from build123d import *

# Parameters (mm, degrees)
SKETCH2_W           = 41
SKETCH2_H           = 41
BOSS_EXTRUDE1_DEPTH = 2
SKETCH3_R           = 2
CUT_EXTRUDE1_DEPTH  = 30.060282173
SKETCH4_R           = 7.5
CUT_EXTRUDE2_DEPTH  = 30.060282173
SKETCH5_W           = 25
SKETCH5_H           = 25
CUT_EXTRUDE3_DEPTH  = 1
CUT_EXTRUDE4_DEPTH  = 30.060282173
SKETCH7_R           = 2
CUT_EXTRUDE5_DEPTH  = 30.060282173
SKETCH8_W           = 25
SKETCH8_H           = 8
SKETCH8_H_2         = 7.957817611
BOSS_EXTRUDE2_DEPTH = 3.5
SKETCH9_R           = 2
CUT_EXTRUDE6_DEPTH  = 30.508473359
BOSS_EXTRUDE3_START = 3.5
SKETCH10_R          = 2
BOSS_EXTRUDE3_DEPTH = 3.5
SKETCH11_R          = 3.5
CUT_EXTRUDE7_DEPTH  = 3.5
SKETCH12_W          = 8
SKETCH12_H          = 2
BOSS_EXTRUDE4_DEPTH = 3.5
SKETCH13_R          = 3.5
CUT_EXTRUDE8_DEPTH  = 3.5
SKETCH14_R          = 3.5
SKETCH14_R_2        = 2
BOSS_EXTRUDE5_DEPTH = 3
SKETCH15_W          = 16
SKETCH15_H          = 8.042182389
SKETCH15_R          = 2
SKETCH15_H_2        = 8
BOSS_EXTRUDE6_DEPTH = 4
SKETCH16_W          = 8
SKETCH16_H          = 25
CUT_EXTRUDE9_DEPTH  = 3.5
SKETCH18_W          = 32.514718626
SKETCH18_H          = 41
CUT_EXTRUDE10_DEPTH = 4
CUT_EXTRUDE12_DEPTH = 30.508473359


with BuildPart() as part:
    # Sketch2 → Boss-Extrude1 (new body)
    with BuildSketch(Plane(origin=(0, 0, 0), x_dir=(1, 0, 0), z_dir=(0, 1, 0))):
        Rectangle(SKETCH2_W, SKETCH2_H)
    extrude(amount=BOSS_EXTRUDE1_DEPTH)

    # Sketch3 → Cut-Extrude1 (cut, through all)
    with BuildSketch(Plane.XZ):
        with Locations(Location((-7.943181907, 8.037155044, 0), (0, 0, 270))):
            Circle(SKETCH3_R)
        with Locations(Location((8.037155044, 7.943181907, 0), (0, 0, 270))):
            Circle(SKETCH3_R)
        with Locations(Location((7.943181907, -8.037155044, 0), (0, 0, 270))):
            Circle(SKETCH3_R)
        with Locations(Location((-8.037155044, -7.943181907, 0), (0, 0, 270))):
            Circle(SKETCH3_R)
    extrude(amount=-CUT_EXTRUDE1_DEPTH, mode=Mode.SUBTRACT)

    # Sketch4 → Cut-Extrude2 (cut, through all)
    with BuildSketch(Plane(origin=(0, 2, 0), x_dir=(1, 0, 0), z_dir=(0, 1, 0))):
        with Locations(Location((0, 0, 0), (0, 0, 270))):
            Circle(SKETCH4_R)
    extrude(amount=-CUT_EXTRUDE2_DEPTH, mode=Mode.SUBTRACT)

    # Sketch5 → Cut-Extrude3 (cut)
    with BuildSketch(Plane.XZ):
        Rectangle(SKETCH5_W, SKETCH5_H)
    extrude(amount=-CUT_EXTRUDE3_DEPTH, mode=Mode.SUBTRACT)

    # Sketch6 → Cut-Extrude4 (cut, through all)
    with BuildSketch(Plane(origin=(0, 2, 0), x_dir=(1, 0, 0), z_dir=(0, 1, 0))):
        Polygon((-20.5, 16.257359313), (-16.257359313, 20.5), (-20.5, 20.5), align=None)
        Polygon((16.257359313, 20.5), (20.5, 16.257359313), (20.5, 20.5), align=None)
        Polygon((20.5, -16.257359313), (16.257359313, -20.5), (20.5, -20.5), align=None)
        Polygon((-16.257359313, -20.5), (-20.5, -16.257359313), (-20.5, -20.5), align=None)
    extrude(amount=-CUT_EXTRUDE4_DEPTH, mode=Mode.SUBTRACT)

    # Sketch7 → Cut-Extrude5 (cut, through all)
    with BuildSketch(Plane.XZ):
        with Locations(Location((-15.5, 15.5, 0), (0, 0, 270))):
            Circle(SKETCH7_R)
        with Locations(Location((15.5, 15.5, 0), (0, 0, 270))):
            Circle(SKETCH7_R)
        with Locations(Location((15.5, -15.5, 0), (0, 0, 270))):
            Circle(SKETCH7_R)
        with Locations(Location((-15.5, -15.5, 0), (0, 0, 270))):
            Circle(SKETCH7_R)
    extrude(amount=-CUT_EXTRUDE5_DEPTH, mode=Mode.SUBTRACT)

    # Sketch8 → Boss-Extrude2 (add)
    with BuildSketch(Plane.XZ):
        with Locations((0, 16.5)):
            Rectangle(SKETCH8_W, SKETCH8_H)
        with Locations((0, -16.478908806)):
            Rectangle(SKETCH8_W, SKETCH8_H_2)
    extrude(amount=BOSS_EXTRUDE2_DEPTH)

    # Sketch9 → Cut-Extrude6 (cut, through all)
    with BuildSketch(Plane.XZ.offset(3.5)):
        with Locations(Location((0, 16.5, 0), (0, 0, 270))):
            Circle(SKETCH9_R)
        with Locations(Location((0, -16.478908806, 0), (0, 0, 270))):
            Circle(SKETCH9_R)
    extrude(amount=-CUT_EXTRUDE6_DEPTH, mode=Mode.SUBTRACT)

    # Sketch10 → Boss-Extrude3 (add)
    # profile 1 of 3: a face of its own
    with BuildSketch(Plane.XZ.offset(BOSS_EXTRUDE3_START)):
        Polygon((-20.5, 16.257359313), (-20.5, 12.5), (-12.5, 12.5), (-12.5, 20.5), (-16.257359313, 20.5), align=None)
        with Locations(Location((-15.5, 15.5, 0), (0, 0, 270))):
            Circle(SKETCH10_R, mode=Mode.SUBTRACT)
    # profile 2 of 3: a face of its own
    with BuildSketch(Plane.XZ.offset(BOSS_EXTRUDE3_START)):
        Polygon((12.5, 12.5), (20.5, 12.5), (20.5, 16.257359313), (16.257359313, 20.5), (12.5, 20.5), align=None)
        with Locations(Location((15.5, 15.5, 0), (0, 0, 270))):
            Circle(SKETCH10_R, mode=Mode.SUBTRACT)
    # profile 3 of 3: a face of its own
    with BuildSketch(Plane.XZ.offset(BOSS_EXTRUDE3_START)):
        Polygon((-20.5, -12.5), (-20.5, -16.257359313), (-16.257359313, -20.5), (16.257359313, -20.5), (20.5, -16.257359313), (20.5, -12.5), (12.5, -12.5), (12.5, -20.457817611), (-12.5, -20.457817611), (-12.5, -12.5), align=None)
        with Locations(Location((-15.5, -15.5, 0), (0, 0, 270))):
            Circle(SKETCH10_R, mode=Mode.SUBTRACT)
        with Locations(Location((15.5, -15.5, 0), (0, 0, 270))):
            Circle(SKETCH10_R, mode=Mode.SUBTRACT)
    extrude(amount=-BOSS_EXTRUDE3_DEPTH)

    # Sketch11 → Cut-Extrude7 (cut)
    with BuildSketch(Plane(origin=(0, 2, 0), x_dir=(1, 0, 0), z_dir=(0, 1, 0))):
        with Locations(Location((-15.5, 15.5, 0), (0, 0, 270))):
            Circle(SKETCH11_R)
        with Locations(Location((15.5, 15.5, 0), (0, 0, 270))):
            Circle(SKETCH11_R)
        with Locations(Location((15.5, -15.5, 0), (0, 0, 270))):
            Circle(SKETCH11_R)
        with Locations(Location((-15.5, -15.5, 0), (0, 0, 270))):
            Circle(SKETCH11_R)
    extrude(amount=-CUT_EXTRUDE7_DEPTH, mode=Mode.SUBTRACT)

    # Sketch12 → Boss-Extrude4 (add)
    with BuildSketch(Plane.XZ):
        with Locations((-16.5, -11.5)):
            Rectangle(SKETCH12_W, SKETCH12_H)
        with Locations((-16.5, 11.5)):
            Rectangle(SKETCH12_W, SKETCH12_H)
        with Locations((16.5, -11.5)):
            Rectangle(SKETCH12_W, SKETCH12_H)
        with Locations((16.5, 11.5)):
            Rectangle(SKETCH12_W, SKETCH12_H)
    extrude(amount=BOSS_EXTRUDE4_DEPTH)

    # Sketch13 → Cut-Extrude8 (cut)
    with BuildSketch(Plane(origin=(0, 2, 0), x_dir=(1, 0, 0), z_dir=(0, 1, 0))):
        with Locations(Location((-15.5, 15.5, 0), (0, 0, 270))):
            Circle(SKETCH13_R)
        with Locations(Location((15.5, 15.5, 0), (0, 0, 270))):
            Circle(SKETCH13_R)
        with Locations(Location((15.5, -15.5, 0), (0, 0, 270))):
            Circle(SKETCH13_R)
        with Locations(Location((-15.5, -15.5, 0), (0, 0, 270))):
            Circle(SKETCH13_R)
    extrude(amount=-CUT_EXTRUDE8_DEPTH, mode=Mode.SUBTRACT)

    # Sketch14 → Boss-Extrude5 (add)
    # profile 1 of 4: a face of its own
    with BuildSketch(Plane(origin=(0, -1.5, 0), x_dir=(1, 0, 0), z_dir=(0, 1, 0))):
        with Locations(Location((-15.5, -15.5, 0), (0, 0, 270))):
            Circle(SKETCH14_R)
        with Locations(Location((-15.5, -15.5, 0), (0, 0, 90))):
            Circle(SKETCH14_R_2, mode=Mode.SUBTRACT)
    # profile 2 of 4: a face of its own
    with BuildSketch(Plane(origin=(0, -1.5, 0), x_dir=(1, 0, 0), z_dir=(0, 1, 0))):
        with Locations(Location((-15.5, 15.5, 0), (0, 0, 270))):
            Circle(SKETCH14_R)
        with Locations(Location((-15.5, 15.5, 0), (0, 0, 90))):
            Circle(SKETCH14_R_2, mode=Mode.SUBTRACT)
    # profile 3 of 4: a face of its own
    with BuildSketch(Plane(origin=(0, -1.5, 0), x_dir=(1, 0, 0), z_dir=(0, 1, 0))):
        with Locations(Location((15.5, 15.5, 0), (0, 0, 270))):
            Circle(SKETCH14_R)
        with Locations(Location((15.5, 15.5, 0), (0, 0, 90))):
            Circle(SKETCH14_R_2, mode=Mode.SUBTRACT)
    # profile 4 of 4: a face of its own
    with BuildSketch(Plane(origin=(0, -1.5, 0), x_dir=(1, 0, 0), z_dir=(0, 1, 0))):
        with Locations(Location((15.5, -15.5, 0), (0, 0, 270))):
            Circle(SKETCH14_R)
        with Locations(Location((15.5, -15.5, 0), (0, 0, 90))):
            Circle(SKETCH14_R_2, mode=Mode.SUBTRACT)
    extrude(amount=BOSS_EXTRUDE5_DEPTH)

    # Sketch15 → Boss-Extrude6 (add)
    # profile 1 of 2: a face of its own
    with BuildSketch(Plane(origin=(0, 2, 0), x_dir=(1, 0, 0), z_dir=(0, 1, 0))):
        with Locations((0, 16.478908806)):
            Rectangle(SKETCH15_W, SKETCH15_H)
        with Locations(Location((0, 16.478908806, 0), (0, 0, 90))):
            Circle(SKETCH15_R, mode=Mode.SUBTRACT)
    # profile 2 of 2: a face of its own
    with BuildSketch(Plane(origin=(0, 2, 0), x_dir=(1, 0, 0), z_dir=(0, 1, 0))):
        with Locations((0, -16.5)):
            Rectangle(SKETCH15_W, SKETCH15_H_2)
        with Locations(Location((0, -16.478908806, 0), (0, 0, 90))):
            Circle(SKETCH15_R, mode=Mode.SUBTRACT)
    extrude(amount=BOSS_EXTRUDE6_DEPTH)

    # Sketch16 → Cut-Extrude9 (cut)
    with BuildSketch(Plane.XZ.offset(3.5)):
        with Locations((-16.5, 0)):
            Rectangle(SKETCH16_W, SKETCH16_H)
        with Locations((16.5, 0)):
            Rectangle(SKETCH16_W, SKETCH16_H)
    extrude(amount=-CUT_EXTRUDE9_DEPTH, mode=Mode.SUBTRACT)

    # Sketch18 → Cut-Extrude10 (cut)
    with BuildSketch(Plane(origin=(0, 6, 0), x_dir=(1, 0, 0), z_dir=(0, 1, 0))):
        Rectangle(SKETCH18_W, SKETCH18_H)
    extrude(amount=-CUT_EXTRUDE10_DEPTH, mode=Mode.SUBTRACT)

    # Sketch19 → Cut-Extrude12 (cut, through all)
    with BuildSketch(Plane(origin=(0, 2, 0), x_dir=(1, 0, 0), z_dir=(0, 1, 0))):
        Polygon((-12, 20.5), (-12, -20.5), (-16.257359313, -20.5), (-20.5, -16.257359313), (-20.5, 16.257359313), (-16.257359313, 20.5), align=None)
    extrude(amount=-CUT_EXTRUDE12_DEPTH, mode=Mode.SUBTRACT)


solid = part.part
Input: part model. Units: mm. Frame: model coordinates. A direction names the side the tool comes from. Give positions to 0.01 mm unless a question says otherwise; leave off trailing zeros. Order: outer loops, then holes, each group sorted by start corner. A loop starts at its lowest first (then second) coordinate and runs counter-clockwise, first axis right, second up.
Q1. Ray query, probe 1 along X at (y, z) = (1.65, 8); probe 2 along Z at (x, y) = (4, 0.8); probe 3 along X at (y, z) = (-1.45, 15.5). Return the intervals inside material, ascending.
Checked values:
probe 1: x = -12 to -9.94, -5.94 to 6.04, 10.04 to 20.5
probe 2: z = -20.5 to -12.5, 12.5 to 20.5
probe 3: x = -12 to -1.73, 1.73 to 13.5, 17.5 to 20.5
Q2. Section B-B on y = -0.6. Output: boundary loops of the cut face in (x, z).
Checked values:
outline: (-12, -20.5) - (16.26, -20.5) - (20.5, -16.26) - (20.5, -12.5) - (-12, -12.5) - close; (-12, 12.5) - (20.5, 12.5) - (20.5, 16.26) - (16.26, 20.5) - (-12, 20.5) - close; hole circle Ø4 at (0, -16.48); hole circle Ø4 at (0, 16.5); hole circle Ø4 at (15.5, -15.5); hole circle Ø4 at (15.5, 15.5)
Q3. Contact query for flat-ended pins moving along their axis: pin 1 Ø1.1 at (y, z) = (0.5, -6) entering from -X; pin 2 Ø1 at (x, z) = (-1, -8.5) entering from -Y; pin 3 Ø4.5 at (x, z) = (15.5, -15.5) entering from +Y; pin 4 Ø2.5 at (x, z) = (16, 1.5) entering from -Y. Output: stop coordinate, or through.
Checked values:
pin 1: stops at x = -12
pin 2: stops at y = 1
pin 3: stops at y = 1.5
pin 4: stops at y = 0
Q4. Section C-C on x = 15.5. Output: boundary loops of the cut face in (y, z).
Checked values:
outline: (-3.5, -20.5) - (2, -20.5) - (2, -19) - (1.5, -19) - (1.5, -17.5) - (-3.5, -17.5) - close; (-3.5, -13.5) - (1.5, -13.5) - (1.5, -12) - (2, -12) - (2, 12) - (1.5, 12) - (1.5, 13.5) - (-3.5, 13.5) - (-3.5, 12.5) - (0, 12.5) - (0, -12.5) - (-3.5, -12.5) - close; (-3.5, 17.5) - (1.5, 17.5) - (1.5, 19) - (2, 19) - (2, 20.5) - (-3.5, 20.5) - close
Q5. Set-up query: faces 4 (the flat face through (6, 1, 6)), 5 (the cylindrical face through (16.55, 1.75, -12.16)), 6 (the cylindrical face through (0.33, 1.507, -7.493)). Return all of +Z, -Z, +X, -X, +Y, -Y with unobstructed straight access to the full face (end or side cutting, diameter ignored); none if empty.
Checked values:
face 4: -X, -Y
face 5: +Y
face 6: +Y, -Y
Q6. Section D-D on x = 11. Output: boundary loops of the cut face in (y, z), and give its area (3 significant figures).
Checked values:
outline: (-3.5, -20.5) - (2, -20.5) - (2, 20.5) - (-3.5, 20.5) - (-3.5, 12.5) - (1, 12.5) - (1, -12.5) - (-3.5, -12.5) - close
area: 113 mm2
Q7. Draft query along X for faces 1 (the flat face through (4, -1, -12.5)), 2 (the flat face through (12.5, 0.5, -0.2)), 3 (the cylindrical face through (-6.35, 1.49, -9.02)). Return one class per face: +X half, -X half, draft (parallel to the pull), parting line (faces both ways), or undercut.
Checked values:
face 1: draft
face 2: -X half
face 3: undercut
Q8. Section A-A on z = 0. Output: boundary loops of the cut face in (x, y).
Checked values:
outline: (-12, 1) - (-7.5, 1) - (-7.5, 2) - (-12, 2) - close; (7.5, 1) - (12.5, 1) - (12.5, 0) - (20.5, 0) - (20.5, 2) - (7.5, 2) - close
